Source: CAD feature listing. Evaluate the final solid. Frame: model axes, mm. A direction names the side the tool comes from. Round coordinates to 2 decimals unless told otherwise and drop trailing zeros. Order: outer loops, then holes, each group sorted by start corner. A loop starts at its lowest first (then second) coordinate and runs counter-clockwise, first axis right, second up. Notation, with made-up numbers: (46.5, 27.25) - (73.5, 27.25) arc R30 ccw to (73.5, 56.25) - close; hole circle Ø3 at (39, 58.5). An arc over 180 degrees is marked (long way). Put each result on its own line as item: value. Start each with the question number.
1) Contact query for a flat-ended pin moving along its axis: P1, Ø11.5, axis at x = 15, z = 0, coming from the +Y side. Output: stop coordinate, or through.
2) Access query for faces 1 (the face through (-30, 6, 0)), 2 (the face through (20, 3, 0)). Directions: +Z, -Z, +X, -X, +Y, -Y. A direction counts if a zero-diameter tool reaches every point of the face in a straight line with its end or side. Return the directions, or none.
3) Section B-B on y = 5.75. Output: boundary loops of the cut face in (x, z), then the cut area to 3 significant figures.
4) Line query: probe 1 along X at (y, z) = (7.75, -1); probe 2 along Z at (x, y) = (-15, 8.5); probe 3 along Z at (x, y) = (15, 1.3). Output: solid intervals per line, ascending. Write a range as [from, to].
5) Section A-A on x = 0. Output: boundary loops of the cut face in (y, z).
6) Section C-C on z = -3.25. Output: boundary loops of the cut face in (x, y), then the cut area to 3 significant figures.
7) Section D-D on z = 0. Output: boundary loops of the cut face in (x, y).
```python
from build123d import *

# Parameters (mm, degrees)
SKETCH_1_W             = 60
SKETCH_1_H             = 30
EXTRUDE_1_DEPTH        = 12
HOLE_WIZARD_M121_D     = 10.2
HOLE_WIZARD_M121_DEPTH = 12


with BuildPart() as part:
    # Эскиз1 → Бобышка-Вытянуть1 (new body)
    with BuildSketch(Plane(origin=(0, 0, 0), x_dir=(1, 0, 0), z_dir=(0, 1, 0))):
        Rectangle(SKETCH_1_W, SKETCH_1_H)
    extrude(amount=EXTRUDE_1_DEPTH)

    # Эскиз2 → Вырез-Повернуть1 (revolve, cut)
    with BuildSketch(Plane.XY):
        Polygon((-22.5, 12), (-22.5, 3), (-19.5, 3), (-19.5, 0), (-15, 0), (-15, 12), align=None)
    cut_revolve_1 = revolve(axis=Axis((-15, 12, 0), (0, -1, 0)), mode=Mode.SUBTRACT)

    # Зеркальное отражение1: Вырез-Повернуть1 across plane
    add(cut_revolve_1.mirror(Plane(origin=(0, 0, 0), x_dir=(0, 0, 1), z_dir=(1, 0, 0))), mode=Mode.SUBTRACT)

    # Отверстие обработанное метчиком M121
    with Locations(Plane(origin=(0, 12, 0), x_dir=(1, 0, 0), z_dir=(0, 1, 0))):
        with Locations((0, 0)):
            Hole(HOLE_WIZARD_M121_D / 2, depth=HOLE_WIZARD_M121_DEPTH)


solid = part.part
```
Answer sheet:
1. P1: y = 3
2. face 1: +Z, -Z, -X, +Y, -Y
2. face 2: +Y
3. outline: (-30, -15) - (30, -15) - (30, 15) - (-30, 15) - close; hole circle Ø15 at (-15, 0); hole circle Ø10.2 at (0, 0); hole circle Ø15 at (15, 0)
3. area: 1,360 mm^2
4. probe 1: [-30, -22.43], [-7.57, -5], [5, 7.57], [22.43, 30]
4. probe 2: [-15, -7.5], [7.5, 15]
4. probe 3: [-15, -4.5], [4.5, 15]
5. outline: (0, -15) - (12, -15) - (12, -5.1) - (0, -5.1) - close; (0, 5.1) - (12, 5.1) - (12, 15) - (0, 15) - close
6. outline: (-30, 0) - (-18.11, 0) - (-18.11, 3) - (-21.76, 3) - (-21.76, 12) - (-30, 12) - close; (-11.89, 0) - (-3.93, 0) - (-3.93, 12) - (-8.24, 12) - (-8.24, 3) - (-11.89, 3) - close; (3.93, 0) - (11.89, 0) - (11.89, 3) - (8.24, 3) - (8.24, 12) - (3.93, 12) - close; (18.11, 0) - (30, 0) - (30, 12) - (21.76, 12) - (21.76, 3) - (18.11, 3) - close
6. area: 345 mm^2
7. outline: (-30, 0) - (-19.5, 0) - (-19.5, 3) - (-22.5, 3) - (-22.5, 12) - (-30, 12) - close; (-10.5, 0) - (-5.1, 0) - (-5.1, 12) - (-7.5, 12) - (-7.5, 3) - (-10.5, 3) - close; (5.1, 0) - (10.5, 0) - (10.5, 3) - (7.5, 3) - (7.5, 12) - (5.1, 12) - close; (19.5, 0) - (30, 0) - (30, 12) - (22.5, 12) - (22.5, 3) - (19.5, 3) - close
